from build123d import *

# Parameters (mm, degrees)
SKETCH_1_W                     = 330
SKETCH_1_H                     = 90
EXTRUDE_1_DEPTH                = 12.5
SKETCH_2_W                     = 9.5
SKETCH_2_H                     = 4
CUT_EXTRUDE_1_DEPTH            = 331
HOLE_WIZARD_M4_1_D             = 4.5
HOLE_WIZARD_M4_1_CSINK_D       = 8.96
HOLE_WIZARD_M4_1_CSINK_ANGLE   = 90
HOLE_WIZARD_M4_1_2_D           = 3.3
HOLE_WIZARD_M4_1_2_CSINK_D     = 4.05
HOLE_WIZARD_M4_1_2_CSINK_ANGLE = 90
FILLET_2_R                     = 2
FILLET_3_R                     = 2


with BuildPart() as part:
    # 草圖1 → 填料-伸長1 (new body)
    with BuildSketch(Plane.XY):
        with Locations((165, 45)):
            Rectangle(SKETCH_1_W, SKETCH_1_H)
    extrude(amount=EXTRUDE_1_DEPTH)

    # 草圖2 → 除料-伸長1 (cut, through all)
    with BuildSketch(Plane.ZY):
        with Locations((7.75, 88)):
            Rectangle(SKETCH_2_W, SKETCH_2_H)
        with Locations((7.75, 2)):
            Rectangle(SKETCH_2_W, SKETCH_2_H)
    extrude(amount=-CUT_EXTRUDE_1_DEPTH, mode=Mode.SUBTRACT)

    # Hole Wizard M4 _1 (through all)
    with Locations(Plane(origin=(0, 0, 0), x_dir=(-1, 0, 0), z_dir=(0, 0, -1))):
        with Locations((-322.5, 70), (-322.5, 20), (-6, 70), (-6, 20)):
            CounterSinkHole(HOLE_WIZARD_M4_1_D / 2, HOLE_WIZARD_M4_1_CSINK_D / 2, counter_sink_angle=HOLE_WIZARD_M4_1_CSINK_ANGLE)

    # Hole Wizard M4 _1 2 (through all)
    with Locations(Plane(origin=(0, 86, 0), x_dir=(1, 0, 0), z_dir=(0, 1, 0))):
        with Locations((30, -9), (120, -9), (210, -9), (300, -9)):
            CounterSinkHole(HOLE_WIZARD_M4_1_2_D / 2, HOLE_WIZARD_M4_1_2_CSINK_D / 2, counter_sink_angle=HOLE_WIZARD_M4_1_2_CSINK_ANGLE)

    # 圓角2
    fillet_2_edges = [part.edges().sort_by_distance(p)[0] for p in [
        (330, 90, 1.5),
        (330, 0, 1.5),
    ]]
    fillet(fillet_2_edges, radius=FILLET_2_R)

    # 圓角3
    fillet_3_edges = [part.edges().sort_by_distance(p)[0] for p in [
        (164, 90, 0),
        (164, 0, 0),
        (330, 45, 0),
    ]]
    fillet(fillet_3_edges, radius=FILLET_3_R)


solid = part.part
For this review, take the finished solid that the model builds, in its own axes (mm). Round coordinates to 2 decimals unless told otherwise and drop trailing zeros. Loops run counter-clockwise (first coordinate to the right, second up) from the corner with the lowest first, then second, coordinate; pieces in that order, holes last. Notation, with made-up numbers: (4, -12) - (32, -12) arc R22 ccw to (32, 2) - close; hole circle Ø10 at (-1.75, 14). An arc over 180 degrees is marked (long way). Put each result on its own line as item: value. Start each with the question number.
1. Insertion check: P1, Ø5, axis at x = 36.5, z = 7.5, coming from the +Y side; P2, Ø3, axis at x = 203, y = 1.5, coming from the +Z side; P3, Ø3, axis at x = 135, z = 8, coming from the -Y side. Each pin has a flat end and moves straight along its axis. Give the tip position at first contact, or say it passes through.
2. Mouldability with a two-part tool opening along Y and no side actions: class faces 1 (the flat face through (162, 46, 0)), 2 (the conical face through (324.75, 20.71, 2.12)), 3 (the flat face through (163, 4, 8)), 4 (the flat face through (163, 86, 8)) as +Y half, -Y half, draft (parallel to the pull), parting line (faces both ways), or undercut.
3. Consider section A-A on x = 65. State the section outline as (y, z) points, plus the area to 3 significant figures.
4. For probe 1 along X at (y, z) = (20, 4.75); probe 2 along Y at (x, z) = (322.5, 10.25); probe 3 along X at (y, z) = (37, 9), list the stretches that pass through material, from the lowest coordinate up. Write a range as [from, to].
Result sheet:
1. P1: y = 86
1. P2: z = 3
1. P3: y = 4
2. face 1: draft
2. face 2: undercut
2. face 3: -Y half
2. face 4: +Y half
3. outline: (0, 2) arc R2 ccw to (2, 0) - (88, 0) arc R2 ccw to (90, 2) - (90, 3) - (86, 3) - (86, 12.5) - (4, 12.5) - (4, 3) - (0, 3) - close
3. area: 1,050 mm^2
4. probe 1: [0, 3.75], [8.25, 320.25], [324.75, 330]
4. probe 2: [4, 17.75], [22.25, 67.75], [72.25, 86]
4. probe 3: [0, 28.35], [31.65, 118.35], [121.65, 208.35], [211.65, 298.35], [301.65, 330]
